```python
from build123d import *

# Parameters (mm, degrees)
SKETCH1_W                       = 20
SKETCH1_H                       = 11.6
BOSS_EXTRUDE1_DEPTH             = 2
SKETCH2_W                       = 10
SKETCH2_H                       = 1.8
BOSS_EXTRUDE2_DEPTH             = 10
FILLET1_R                       = 5
F_4_0MM_DOWEL_HOLE1_D           = 4
F_4_0MM_DOWEL_HOLE1_CSINK_D     = 4.05
F_4_0MM_DOWEL_HOLE1_CSINK_ANGLE = 90
F_2_0MM_DOWEL_HOLE1_D           = 2
F_2_0MM_DOWEL_HOLE1_CSINK_D     = 2.05
F_2_0MM_DOWEL_HOLE1_CSINK_ANGLE = 90
FILLET2_R                       = 2
FILLET3_R                       = 1


with BuildPart() as part:
    # Sketch1 → Boss-Extrude1 (new body)
    with BuildSketch(Plane(origin=(0, 0, 0), x_dir=(0, 1, 0), z_dir=(0, 0, 1))):
        Rectangle(SKETCH1_W, SKETCH1_H)
    extrude(amount=-BOSS_EXTRUDE1_DEPTH)

    # Sketch2 → Boss-Extrude2 (add)
    with BuildSketch(Plane(origin=(0, 0, 0), x_dir=(0, 1, 0), z_dir=(0, 0, 1))):
        with Locations((0, 4.9)):
            Rectangle(SKETCH2_W, SKETCH2_H)
        with Locations((0, -4.9)):
            Rectangle(SKETCH2_W, SKETCH2_H)
    extrude(amount=BOSS_EXTRUDE2_DEPTH)

    # Fillet1
    fillet1_edges = [part.edges().sort_by_distance(p)[0] for p in [
        (4.9, 5, 10),
        (4.9, -5, 10),
        (-4.9, 5, 10),
        (-4.9, -5, 10),
    ]]
    fillet(fillet1_edges, radius=FILLET1_R - 0.0001)  # a hair under: the kernel refuses the full size

    # Ø4.0mm Dowel Hole1 (through all)
    with Locations(Plane.YZ.offset(5.8)):
        with Locations((0, 5)):
            CounterSinkHole(F_4_0MM_DOWEL_HOLE1_D / 2, F_4_0MM_DOWEL_HOLE1_CSINK_D / 2, counter_sink_angle=F_4_0MM_DOWEL_HOLE1_CSINK_ANGLE)

    # Ø2.0mm Dowel Hole1 (through all)
    with Locations(Plane(origin=(0, 0, 0), x_dir=(0, 1, 0), z_dir=(0, 0, 1))):
        with Locations((7.5, -3), (-7.5, 3), (-7.5, -3), (7.5, 3)):
            CounterSinkHole(F_2_0MM_DOWEL_HOLE1_D / 2, F_2_0MM_DOWEL_HOLE1_CSINK_D / 2, counter_sink_angle=F_2_0MM_DOWEL_HOLE1_CSINK_ANGLE)

    # Fillet2
    fillet2_edges = [part.edges().sort_by_distance(p)[0] for p in [
        (-5.8, -10, -1),
        (-5.8, 10, -1),
        (5.8, 10, -1),
        (5.8, -10, -1),
    ]]
    fillet(fillet2_edges, radius=FILLET2_R)

    # Fillet3
    fillet3_edges = [part.edges().sort_by_distance(p)[0] for p in [
        (-4.9, -5, 0),
        (-4.9, 5, 0),
        (4.9, -5, 0),
        (4.9, 5, 0),
    ]]
    fillet(fillet3_edges, radius=FILLET3_R)


solid = part.part
```
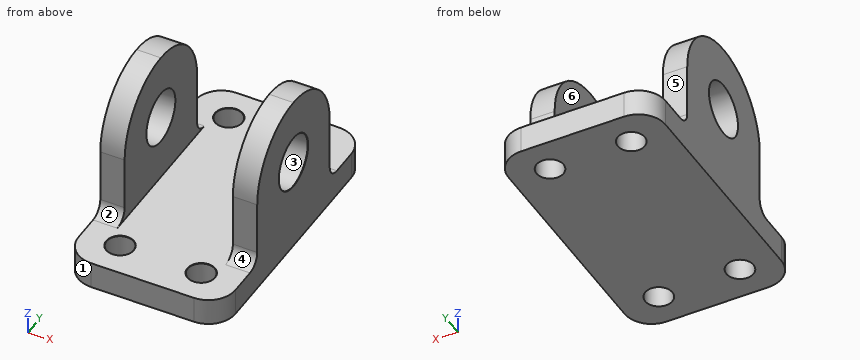
Could you check a few things on this model? Use its own coordinates, in mm. Face numbers are marked on the shaded views. A direction names the side the tool comes from. Round coordinates to 2 decimals unless told otherwise and drop trailing zeros. Loops run counter-clockwise (first coordinate to the right, second up) from the corner with the lowest first, then second, coordinate; pieces in that order, holes last. Notation, with made-up numbers: (-28, -31.75) - (25, -31.75) arc R13 ccw to (25, -21.75) - close; hole circle Ø4 at (57.25, 3.25). An arc over 180 degrees is marked (long way). Answer in a Markdown table with one row per item. Add a question column.
(1) If we section it at C-C (y = 7.5): Please give me the cut outline in (x, z) (3 decimals).
(2) If we section it at B-B (z = 1.5): Please give me the cut outline in (x, y), plus the area to 3 significant figures.
(3) I'm going to push flat-ended pins straight in: pin 1 (3 mm diameter, centred on x = -3, y = -7.5, fed in from -Z); pin 2 (2 mm diameter, centred on x = -5, z = 3, fed in from -Y); pin 3 (0.9 mm diameter, centred on x = 5, z = 3.5, fed in from +Y). Where does each tip first touch, or does it pass through?
(4) If we mould it in two halves opening along Z, with no side actions, what happens to the marked faces 1, 2 and 3? For each: pulls with the +Z half, pulls with the -Z half, needs draft (parallel to the pull), parting line crosses it, or undercut.
(5) I need wall thicknesses on line 1 along X through (y, z) = (7.5, -1.2); line 2 along X through (y, z) = (-0.75, 8); line 3 along Y through (x, z) = (4.7, 5). Which ranges of each line are inside material? Lowest first, please.
(6) If we section it at A-A (x = 3): Please give me the cut outline in (y, z) (3 decimals).
(7) For the marked faces 4, 5 and 6, which set-ups out of +Z, -Z, +X, -X, +Y, -Y let a thin tool reach every point of the face, with its end or its side?
(8) If we section it at D-D (z = 6.75): State how many separate pieces and enclosed holes the cut face has, plus the area to 3 significant figures.
Model answer:
| question | item | result |
|---|---|---|
| 1 | outline | (-5.8, -2) - (-4, -2) - (-4, -0.025) - (-4.025, 0) - (-5.8, 0) - close; (-2, -2) - (2, -2) - (2, -0.025) - (1.975, 0) - (-1.975, 0) - (-2, -0.025) - close; (4, -2) - (5.8, -2) - (5.8, 0) - (4.025, 0) - (4, -0.025) - close |
| 2 | outline | (-5.8, -5) - (-4, -5) - (-4, 5) - (-5.8, 5) - close; (4, -5) - (5.8, -5) - (5.8, 5) - (4, 5) - close |
| 2 | area | 36.0 mm² |
| 3 | pin 1 | stops at z = -2 |
| 3 | pin 2 | stops at y = -5 |
| 3 | pin 3 | stops at y = 5 |
| 4 | face 1 | needs draft |
| 4 | face 2 | pulls with the +Z half |
| 4 | face 3 | undercut |
| 5 | line 1 | x = -5.8 to -4, -2 to 2, 4 to 5.8 |
| 5 | line 2 | x = -5.8 to -4, 4 to 5.8 |
| 5 | line 3 | y = -5 to -2, 2 to 5 |
| 6 | outline | (-10, -2) - (-8.5, -2) - (-8.5, -0.025) - (-8.525, 0) - (-10, 0) - close; (-6.5, -2) - (6.5, -2) - (6.5, -0.025) - (6.475, 0) - (-6.475, 0) - (-6.5, -0.025) - close; (8.5, -2) - (10, -2) - (10, 0) - (8.525, 0) - (8.5, -0.025) - close |
| 7 | face 4 | +Z, +X, -X, -Y |
| 7 | face 5 | +Z, +X, -X, +Y |
| 7 | face 6 | +Z, +Y, -Y |
| 8 | separate pieces | 4 |
| 8 | enclosed holes | 0 |
| 8 | area | 26.8 mm² |
